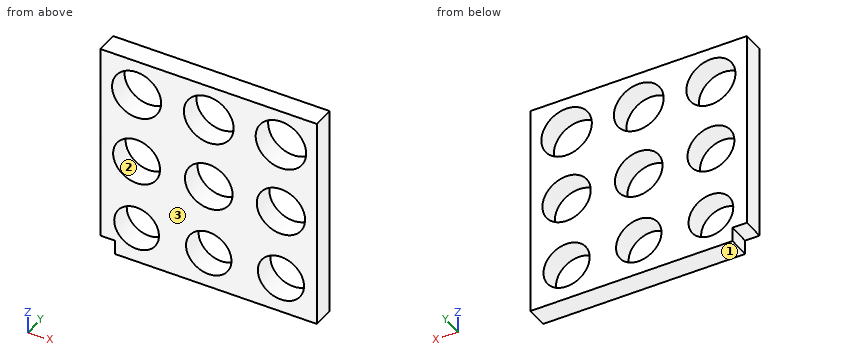
```python
from build123d import *

# Parameters (mm, degrees)
SKETCH1_W           = 15
SKETCH1_H           = 15
BOSS_EXTRUDE1_DEPTH = 1.5
SKETCH2_R           = 1.55
SKETCH2_R_2         = 1.575
SKETCH2_R_3         = 1.6
SKETCH2_R_4         = 1.625
SKETCH2_R_5         = 1.65
SKETCH2_R_6         = 1.675
SKETCH2_R_7         = 1.7
SKETCH2_R_8         = 1.725
SKETCH2_R_9         = 1.75
CUT_EXTRUDE1_DEPTH  = 10
SKETCH4_W           = 1
SKETCH4_H           = 1
CUT_EXTRUDE2_DEPTH  = 10


with BuildPart() as part:
    # Sketch1 → Boss-Extrude1 (new body)
    with BuildSketch(Plane(origin=(0, 0, 0), x_dir=(1, 0, 0), z_dir=(0, 1, 0))):
        Rectangle(SKETCH1_W, SKETCH1_H)
    extrude(amount=BOSS_EXTRUDE1_DEPTH)

    # Sketch2 → Cut-Extrude1 (cut)
    with BuildSketch(Plane(origin=(0, 1.5, 0), x_dir=(1, 0, 0), z_dir=(0, 1, 0))):
        with Locations(Location((-5, 5, 0), (0, 0, 270))):
            Circle(SKETCH2_R)
        with Locations(Location((0, 5, 0), (0, 0, 270))):
            Circle(SKETCH2_R_2)
        with Locations(Location((5, 5, 0), (0, 0, 270))):
            Circle(SKETCH2_R_3)
        with Locations(Location((-5, 0, 0), (0, 0, 270))):
            Circle(SKETCH2_R_4)
        with Locations(Location((0, 0, 0), (0, 0, 270))):
            Circle(SKETCH2_R_5)
        with Locations(Location((5, 0, 0), (0, 0, 270))):
            Circle(SKETCH2_R_6)
        with Locations(Location((-5, -5, 0), (0, 0, 270))):
            Circle(SKETCH2_R_7)
        with Locations(Location((0, -5, 0), (0, 0, 270))):
            Circle(SKETCH2_R_8)
        with Locations(Location((5, -5, 0), (0, 0, 270))):
            Circle(SKETCH2_R_9)
    extrude(amount=-CUT_EXTRUDE1_DEPTH, mode=Mode.SUBTRACT)

    # Sketch4 → Cut-Extrude2 (cut)
    with BuildSketch(Plane(origin=(0, 1.5, 0), x_dir=(1, 0, 0), z_dir=(0, 1, 0))):
        with Locations((-7, 7)):
            Rectangle(SKETCH4_W, SKETCH4_H)
    extrude(amount=-CUT_EXTRUDE2_DEPTH, mode=Mode.SUBTRACT)


solid = part.part
```
The model under review builds one solid part; all positions refer to its coordinate system, in mm. Face numbers are marked on the shaded views. Round coordinates to 2 decimals unless told otherwise and drop trailing zeros. Order: outer loops, then holes, each group sorted by start corner. A loop starts at its lowest first (then second) coordinate and runs counter-clockwise, first axis right, second up. Notation, with made-up numbers: M 76.25,84.5 L 123.25,84.5 A33 cw 123.25,123.5 Z; hole C 59,49.5 d5. An arc over 180 degrees is marked long. Use a Markdown table: item, result.
1) Wall thickness on line 1 along X through (y, z) = (0.6, 5) (3 decimals); line 2 along X through (y, z) = (0.8, 0) (3 decimals): over which ranges is each line inside the solid? List them lowest first. Write a range as [from, to].
Report:
| item | result |
|---|---|
| line 1 | [-7.5, -6.7], [-3.3, -1.725], [1.725, 3.25], [6.75, 7.5] |
| line 2 | [-7.5, -6.625], [-3.375, -1.65], [1.65, 3.325], [6.675, 7.5] |
2) Consider section B-B (x = 0). Write out the cut boundary in (y, z) (3 decimals), then the cut area to 3 significant figures.
Report:
| item | result |
|---|---|
| outline | M 0,-7.5 L 1.5,-7.5 L 1.5,-6.575 L 0,-6.575 Z; M 0,-3.425 L 1.5,-3.425 L 1.5,-1.65 L 0,-1.65 Z; M 0,1.65 L 1.5,1.65 L 1.5,3.275 L 0,3.275 Z; M 0,6.725 L 1.5,6.725 L 1.5,7.5 L 0,7.5 Z |
| area | 7.65 mm^2 |
3) Draft analysis for pull direction Z (two halves, no side actions). For the marked faces 1, 2 and 3, state which applies: released by +Z, released by -Z, zero draft, split by the parting line, or undercut.
Report:
| item | result |
|---|---|
| face 1 | released by -Z |
| face 2 | undercut |
| face 3 | zero draft |
4) Consider section C-C (y = 0.75). Give the number of separate pieces and of enclosed holes in the cut face, then the cut area to 3 significant figures.
Report:
| item | result |
|---|---|
| separate pieces | 1 |
| enclosed holes | 9 |
| area | 147 mm^2 |
5) Consider section A-A (z = -5). Write out the cut boundary in (x, y) (3 decimals), then the cut area to 4 significant figures.
Report:
| item | result |
|---|---|
| outline | M -7.5,0 L -6.55,0 L -6.55,1.5 L -7.5,1.5 Z; M -3.45,0 L -1.575,0 L -1.575,1.5 L -3.45,1.5 Z; M 1.575,0 L 3.4,0 L 3.4,1.5 L 1.575,1.5 Z; M 6.6,0 L 7.5,0 L 7.5,1.5 L 6.6,1.5 Z |
| area | 8.325 mm^2 |
6) Insertion check: pin 1 (5 mm diameter, centred on x = 6, z = 5, fed in from +Y); pin 2 (0.8 mm diameter, centred on x = -7, y = 1, fed in from -Z). Each pin has a flat end and moves straight along its axis. Give the tip position at first contact, or say it passes through.
Report:
| item | result |
|---|---|
| pin 1 | y = 1.5 |
| pin 2 | z = -6.5 |
